Build history of the part. All positions in model axes, mm. Round coordinates to 2 decimals unless told otherwise and drop trailing zeros. Write each loop counter-clockwise with the first axis right and the second up, starting at its lowest first coordinate (ties: lowest second). Pieces come first, ordered by that corner, then holes. Notation, with made-up numbers: (52.25, -39.75) - (57.25, -39.75) arc R23 ccw to (57.25, -24.75) - close; hole circle Ø3 at (-31.5, -5). An arc over 180 degrees is marked (long way). Write each question's results on one line, items separated by ' | '.
from build123d import *

# Parameters (mm, degrees)
F0_W     = 20
F0_H     = 180
F1_DEPTH = 5
F2_R     = 3
F3_DEPTH = 5.001
F5_D     = 6
F7_D     = 6
F8_SIZE  = 0.5
F9_R     = 4


with BuildPart() as f1:
    # F0 (on Front) → F1 (new body)
    with BuildSketch(Plane.XZ):
        with Locations((10, 90)):
            Rectangle(F0_W, F0_H)
    extrude(amount=F1_DEPTH)

    # F2 (on face) → F3 (cut, through all)
    with BuildSketch(Plane.XZ.offset(5)):
        with Locations((10, 170)):
            Circle(F2_R)
    extrude(amount=-F3_DEPTH, mode=Mode.SUBTRACT)

    # F5 (through all)
    with Locations(Plane.XZ.offset(5)):
        with Locations((10, 70)):
            Hole(F5_D / 2)

    # F7 (through all)
    with Locations(Plane.XZ.offset(5)):
        with Locations((10, 10), (10, 20)):
            Hole(F7_D / 2)

    # F8
    f8_edges = [f1.edges().sort_by_distance(p)[0] for p in [
        (7, -5, 170),
        (7, 0, 170),
        (7, 0, 10),
        (7, 0, 20),
        (7, 0, 70),
        (7, -5, 10),
        (7, -5, 20),
        (7, -5, 70),
    ]]
    chamfer(f8_edges, length=F8_SIZE)

    # F9
    f9_edges = [f1.edges().sort_by_distance(p)[0] for p in [
        (20, -2.5, 180),
        (0, -2.5, 180),
    ]]
    fillet(f9_edges, radius=F9_R)


solid = f1.part
(1) Drill centre lines: probe 1 along Z at (x, y) = (10, -2.85); probe 2 along Z at (x, y) = (12, -0.8); probe 3 along X at (y, z) = (-2.95, 170.5). Where is each one in solid material? Low to high. Write a range as [from, to].
Worked answers:
probe 1: z = [0, 7], [13, 17], [23, 67], [73, 167], [173, 180] | probe 2: z = [0, 7.76], [12.24, 17.76], [22.24, 67.76], [72.24, 167.76], [172.24, 180] | probe 3: x = [0, 7.04], [12.96, 20]
(2) Slice it at A-A, the plane y = -2.75. Write the cut outline in (x, z).
Worked answers:
outline: (0, 0) - (20, 0) - (20, 176) arc R4 ccw to (16, 180) - (4, 180) arc R4 ccw to (0, 176) - close; hole circle Ø6 at (10, 10); hole circle Ø6 at (10, 20); hole circle Ø6 at (10, 70); hole circle Ø6 at (10, 170)
(3) Two-plate mould, pull along Z, no slides. Class faces 1 (the flat face through (10, -2, 0)), 2 (the cylindrical face through (18.797, -2.535, 178.859)), 3 (the cylindrical face through (10.65, -2.47, 67.07)), 4 (the flat face through (20, -2, 87)): released by +Z, released by -Z, zero draft, split by the parting line, or undercut.
Worked answers:
face 1: released by -Z | face 2: released by +Z | face 3: undercut | face 4: zero draft
(4) Slice it at B-B, the plane z = 10. Write the cut outline in (x, y).
Worked answers:
outline: (0, -5) - (6.5, -5) - (7, -4.5) - (7, -0.5) - (6.5, 0) - (0, 0) - close; (13, -4.5) - (13.5, -5) - (20, -5) - (20, 0) - (13.5, 0) - (13, -0.5) - close
